Could you check a few things on this model? Use its own coordinates, in mm. A direction names the side the tool comes from. Round coordinates to 2 decimals unless told otherwise and drop trailing zeros. Loops run counter-clockwise (first coordinate to the right, second up) from the corner with the lowest first, then second, coordinate; pieces in that order, holes last. Notation, with made-up numbers: (4, 50) - (50, 50) arc R12 cw to (50, 64) - close; hole circle Ø10 at (-20.5, 26.5). An arc over 180 degrees is marked (long way). Answer as CSV lines item,"result". Start each with the question number.
1) Suppose I cut it at C-C, the plane y = 1.25. Write out the boundary of the cut face in (x, z).
2) Please list where these lines run through material, in increasing order: line 1 along Z through (x, y) = (0, 6.9); line 2 along Y through (x, z) = (-13, 11.5); line 3 along X through (y, z) = (4.5, -5.5).
3) Which directions (+Z, -Z, +X, -X, +Y, -Y) give clear straight access to the entire face, cutting with the end or side of a thin tool? Please do faces 1 (the face through (17, 5.5, 11)), 2 (the face through (-1, 5.8, 12)), 3 (the face through (-0.358, 6.486, -20.227)).
4) We'd pull the mould along X, two halves only. Please class faces 4 (the face through (-9.66, 2.86, -6.49)), 5 (the face through (4, 2.5, -14)), 6 (the face through (15.65, 3.98, 5.37)): pulls with the +X half, pulls with the -X half, needs draft (parallel to the pull), parting line crosses it, or undercut.
5) I'm going to push flat-ended pins straight in: pin 1 Ø2 at (x, z) = (0.5, 11.5) entering from +Y; pin 2 Ø3.5 at (x, z) = (-1.5, -17.5) entering from -Y; pin 3 Ø9 at (x, z) = (-15.16, 8.75) entering from -Y; pin 4 Ø3.5 at (x, z) = (0, -17.5) entering from +Y. Where does each tip first touch, or does it pass through?
6) Suppose I cut it at B-B, the plane y = 6.5. Write out the boundary of the cut face in (x, z).
7) Suppose I cut it at A-A, the plane z = 0. Write out the boundary of the cut face in (x, y).
```python
from build123d import *

# Parameters (mm, degrees)
SKETCH1_R           = 22
SKETCH1_R_2         = 2.75
SKETCH1_R_3         = 7.5
SKETCH1_R_4         = 1
BOSS_EXTRUDE1_DEPTH = 7.5
SKETCH2_R           = 22
SKETCH2_R_2         = 13.5
CUT_EXTRUDE1_DEPTH  = 2.5
FILLET2_R           = 1
CUT_EXTRUDE2_DEPTH  = 1.7
CUT_EXTRUDE3_DEPTH  = 3


with BuildPart() as part:
    # Sketch1 → Boss-Extrude1 (new body)
    with BuildSketch(Plane(origin=(0, 0, 0), x_dir=(1, 0, 0), z_dir=(0, 1, 0))):
        Circle(SKETCH1_R)
        with Locations((0, 17.5)):
            Circle(SKETCH1_R_2, mode=Mode.SUBTRACT)
        with Locations((-15.155444566, -8.75)):
            Circle(SKETCH1_R_2, mode=Mode.SUBTRACT)
        with Locations((15.155444566, -8.75)):
            Circle(SKETCH1_R_2, mode=Mode.SUBTRACT)
        Circle(SKETCH1_R_3, mode=Mode.SUBTRACT)
        with Locations((-9.526279442, 5.5)):
            Circle(SKETCH1_R_4, mode=Mode.SUBTRACT)
        with Locations((9.526279442, 5.5)):
            Circle(SKETCH1_R_4, mode=Mode.SUBTRACT)
        with Locations((0, -11)):
            Circle(SKETCH1_R_4, mode=Mode.SUBTRACT)
    extrude(amount=BOSS_EXTRUDE1_DEPTH)

    # Sketch2 → Cut-Extrude1 (cut)
    with BuildSketch(Plane.XZ):
        Circle(SKETCH2_R)
        Circle(SKETCH2_R_2, mode=Mode.SUBTRACT)
    extrude(amount=-CUT_EXTRUDE1_DEPTH, mode=Mode.SUBTRACT)

    # Fillet2
    fillet2_edges = [part.edges().sort_by_distance(p)[0] for p in [
        (-22, 2.5, 0),
    ]]
    fillet(fillet2_edges, radius=FILLET2_R)

    # Sketch4 → Cut-Extrude2 (cut)
    with BuildSketch(Plane(origin=(0, 7.5, 0), x_dir=(1, 0, 0), z_dir=(0, 1, 0))):
        Polygon((8.157191191, 3.640179929), (10.452386744, 3.384424759), (11.821474995, 5.24424483), (10.895367692, 7.359820071), (8.600172139, 7.615575241), (7.231083889, 5.75575517), align=None)
        Polygon((-1.369088251, -12.859820071), (0.926107302, -13.115575241), (2.295195553, -11.25575517), (1.369088251, -9.140179929), (-0.926107302, -8.884424759), (-2.295195553, -10.74424483), align=None)
        Polygon((-10.895367692, 3.640179929), (-8.600172139, 3.384424759), (-7.231083889, 5.24424483), (-8.157191191, 7.359820071), (-10.452386744, 7.615575241), (-11.821474995, 5.75575517), align=None)
    extrude(amount=-CUT_EXTRUDE2_DEPTH, mode=Mode.SUBTRACT)

    # Sketch5 → Cut-Extrude3 (cut)
    with BuildSketch(Plane.XZ.offset(-2.5)):
        Polygon((12.687667108, 11.82566379), (11.257952861, 8.150673926), (13.725730319, 5.075010135), (17.623222024, 5.67433621), (19.052936271, 9.349326074), (16.585158813, 12.424989865), align=None)
        Polygon((-18.145928854, 11.320337927), (-18.876664651, 7.445333601), (-15.886180363, 4.874995674), (-12.164960279, 6.179662073), (-11.434224481, 10.054666399), (-14.424708769, 12.625004326), align=None)
        Polygon((-3.240770937, -15.253438836), (-3.565964508, -19.183309377), (-0.325193571, -21.429870542), (3.240770937, -19.746561164), (3.565964508, -15.816690623), (0.325193571, -13.570129458), align=None)
    extrude(amount=-CUT_EXTRUDE3_DEPTH, mode=Mode.SUBTRACT)


solid = part.part
```
Filled sheet:
1,outline,"circle Ø27 at (0, 0); hole circle Ø2 at (-9.53, -5.5); hole circle Ø15 at (0, 0); hole circle Ø2 at (0, 11); hole circle Ø2 at (9.53, -5.5)"
2,line 1,"-22 to -20.25, -14.75 to -7.5, 7.5 to 8.99, 13.01 to 22"
2,line 2,"2.5 to 7.5"
2,line 3,"-21.3 to -10.53, -8.53 to -5.1, 5.1 to 8.53, 10.53 to 21.3"
3,face 1,"-Y"
3,face 2,"+Y"
3,face 3,"+Y, -Y"
4,face 4,"undercut"
4,face 5,"needs draft"
4,face 6,"undercut"
5,pin 1,"y = 5.8"
5,pin 2,"y = 5.5"
5,pin 3,"y = 0"
5,pin 4,"through"
6,outline,"circle Ø44 at (0, 0); hole circle Ø5.5 at (-15.16, 8.75); hole (-11.82, -5.76) - (-10.45, -7.62) - (-8.16, -7.36) - (-7.23, -5.24) - (-8.6, -3.38) - (-10.9, -3.64) - close; hole circle Ø15 at (0, 0); hole circle Ø5.5 at (0, -17.5); hole (-2.3, 10.74) - (-0.93, 8.88) - (1.37, 9.14) - (2.3, 11.26) - (0.93, 13.12) - (-1.37, 12.86) - close; hole (7.23, -5.76) - (8.6, -7.62) - (10.9, -7.36) - (11.82, -5.24) - (10.45, -3.38) - (8.16, -3.64) - close; hole circle Ø5.5 at (15.16, 8.75)"
7,outline,"(-22, 3.5) arc R1 ccw to (-21, 2.5) - (-13.5, 2.5) - (-13.5, 0) - (-7.5, 0) - (-7.5, 7.5) - (-22, 7.5) - close; (7.5, 0) - (13.5, 0) - (13.5, 2.5) - (21, 2.5) arc R1 ccw to (22, 3.5) - (22, 7.5) - (7.5, 7.5) - close"
